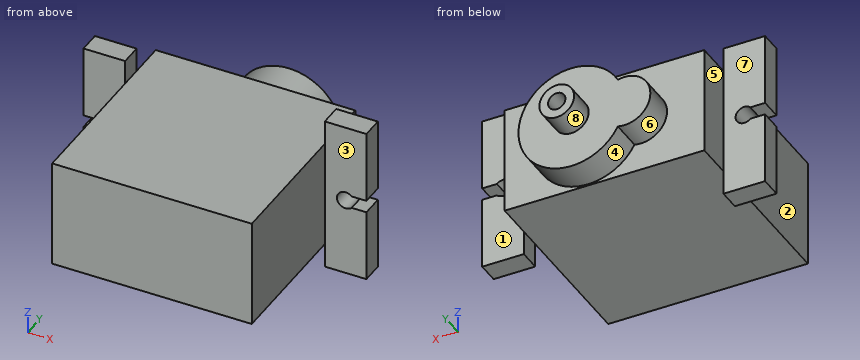
Autodesk Inventor part; units mm, degrees
ref_plane "Work Plane3" through (-11.5, 0, 0) normal (1, 0, 0) x (0, 1, 0)
ref_plane "Work Plane4" through (0, 5, 0) normal (0, 1, 0) x (-1, 0, 0)
ref_plane "Work Plane5" through (0, 0, 6.25) normal (0, 0, 1) x (1, 0, 0)
sketch "Sketch1" plane through (0, 0, 0) normal (0, 1, 0) x (-1, 0, 0)
  line L0 (11.5, -6.25) -> (-11.5, -6.25)
  line L1 (-11.5, -6.25) -> (-11.5, 6.25)
  line L2 (-11.5, 6.25) -> (11.5, 6.25)
  line L3 (11.5, 6.25) -> (11.5, -6.25)
  line L4 (11.5, -6.25) -> (-11.5, 6.25) construction
  line L5 (-11.5, -6.25) -> (11.5, 6.25) construction
  point P0 (0, 0)
  dimension "d0" = 23
  dimension "d1" = 12.5
extrude "Extrusion1" add sketch "Sketch1" along normal mid plane 22.7
ref_plane "Work Plane3" through (-11.5, 0, 0) normal (1, 0, 0) x (0, 1, 0)
ref_plane "Work Plane2" through (11.5, 0, 0) normal (1, 0, 0) x (0, 1, 0)
ref_plane "Work Plane4" through (0, 5, 0) normal (0, 1, 0) x (-1, 0, 0)
ref_plane "Work Plane5" through (0, 0, 6.25) normal (0, 0, 1) x (1, 0, 0)
sketch "Sketch2" plane through (11.5, -11.35, -6.25) normal (1, 0, 0) x (0, 0, -1)
  line L0 (0, 0) -> (-12.5, 0)
  line L1 (-12.5, 0) -> (-12.5, 16)
  line L2 (-12.5, 0) -> (-12.5, 22.7)
  line L3 (-12.5, 16) -> (-15.3, 16)
  line L4 (-15.3, 16) -> (-15.3, 18.5)
  line L5 (-15.3, 18.5) -> (0, 18.5)
  line L6 (0, 18.5) -> (2.8, 18.5)
  line L7 (2.8, 18.5) -> (2.8, 16)
  line L8 (2.8, 16) -> (-12.5, 16)
  point P0 (-6.25, 11.35)
  dimension "d8" = 16
  dimension "d9" = 2.8
  dimension "d10" = 2.5
  dimension "d11" = 2.8
extrude "Extrusion2" add sketch "Sketch2" along normal blind 4.8
mirror "Mirror1" about plane through (0, 0, 0) normal (1, 0, 0) of "Extrusion2"
ref_plane "Work Plane6" through (0, 11, 0) normal (0, 1, 0) x (-1, 0, 0)
sketch "Sketch3" plane through (0, 11, 0) normal (0, 1, 0) x (-1, 0, 0)
  line L0 (-12.5008, 0) -> (-1.9008, 0)
  arc A0 (3.4585, 2.9134) -> (3.4585, -2.9134) centre (-1.9008, 0) ccw
  circle A1 centre (-1.9008, 0) radius 1
  arc A2 (3.4585, -2.9134) -> (3.4585, 2.9134) centre (4.1992, 0) ccw
  point P0 (0, 0)
  dimension "d15" = 10.6
  dimension "d16" = 12.2
  dimension "d17" = 2
extrude "Extrusion3" add sketch "Sketch3" along normal blind 4
sketch "Sketch4" plane through (0, 15, 0) normal (0, 1, 0) x (1, 0, 0)
  circle A0 centre (1.9008, 0) radius 1
  circle A1 centre (1.9008, 0) radius 2
  point P0 (0, 0)
  dimension "d20" = 4
extrude "Extrusion4" add sketch "Sketch4" along normal blind 3.2 contours A0 | A1
sketch "Sketch5" plane through (1.9008, 18.2, 0) normal (0, 1, 0) x (1, 0, 0)
  circle A0 centre (0, 0) radius 1
  circle A1 centre (0, 0) radius 1
  point P0 (-1.9008, 0)
  dimension "d28" = 2
extrude "Extrusion5" cut sketch "Sketch5" against normal blind 3.2
sketch "Sketch6" plane through (11.5, 7.15, -6.25) normal (0, 1, 0) x (1, 0, 0)
  circle A0 centre (-9.5992, -6.25) radius 1
  line L0 (-9.5992, -6.25) -> (1.4, -6.25)
  line L1 (4.8, -15.3) -> (4.8, 2.8)
  line L2 (0, -12.5) -> (0, 0)
  line L3 (0, -6.25) -> (4.8, -6.25)
  arc A1 (3.1037, -5.5395) -> (3.1037, -6.9605) centre (2.4, -6.25) ccw
  line L4 (2.4, -5.25) -> (2.4, -5.25)
  line L5 (3.1037, -5.5395) -> (4.8, -5.5395)
  line L6 (3.1037, -6.9605) -> (4.8, -6.9605)
  line L7 (4.8, -6.9605) -> (4.8, -5.5395)
  point P0 (-11.5, -6.25)
  dimension "d25" = 2
extrude "Extrusion6" cut sketch "Sketch6" against normal blind 2.5 contours A1 L5 L1 L3 | L3 L1 L6 A1
mirror "Mirror2" about plane through (0, 0, 0) normal (1, 0, 0) of "Extrusion6"
properties part number "Motor"
Build history of the part. All positions in model axes, mm. Face numbers are marked on the shaded views. A direction names the side the tool comes from. Coordinates: 2 decimals unless noted, no trailing zeros. Order: outer loops, then holes, each group sorted by start corner. A loop starts at its lowest first (then second) coordinate and runs counter-clockwise, first axis right, second up. Notation, with made-up numbers: M -24,-19 L -5,-19 A30 ccw -5,17 Z; hole C -20.75,12.5 d1. An arc over 180 degrees is marked long. One line per question, with ' | ' between items. Start each with the question number.
Q1. Saw through at A-A (z = 8). List the corners of the cut face in (x, y), then the cut area to 3 significant figures.
Q2. Saw through at C-C (z = 0). List the corners of the cut face in (x, y), then the cut area to 3 significant figures.
Q3. Flat gauge pins, fed straight in: pin 1 Ø8 at (x, z) = (-5.5, 4.5) entering from +Y; pin 2 Ø3 at (y, z) = (2.5, -3.5) entering from -X; pin 3 Ø8 at (x, z) = (-13, -4) entering from +Y. Where does each tip first touch, or does it go through?
Q4. 3-axis set-ups, long thin cutter, end or side, ignore diameter. For the marked faces 1, 2, 3, 4 and 5: which of +Z, -Z, +X, -X, +Y, -Y reach the whole face in a straight line?
Q5. Probe L1, parallel to Z at x = 13.9, y = 6.5; L2, parallel to Y at x = 12, z = -5.5; L3, parallel to Y at x = 10.5, z = 5.5. List the from-to ranges inside material, lowest first. Write a range as from..to.
Q6. Two-plate mould, pull along X, no slides. Class the marked faces 6, 7 and 8: +X half, -X half, draft (parallel to the pull), parting line (faces both ways), or undercut.
Q7. Saw through at B-B (x = -13.9). List the corners of the cut face in (y, z), then the cut area to 4 significant figures.
Q8. Saw through at D-D (x = -1.5). List the corners of the cut face in (y, z).
Check values:
1) outline: M -16.3,4.65 L -11.5,4.65 L -11.5,7.15 L -16.3,7.15 Z; M 11.5,4.65 L 16.3,4.65 L 16.3,7.15 L 11.5,7.15 Z | area: 24.0 mm2
2) outline: M -12.9,4.65 L -11.5,4.65 L -11.5,-11.35 L 11.5,-11.35 L 11.5,4.65 L 12.9,4.65 L 12.9,7.15 L 11.5,7.15 L 11.5,11.35 L 8,11.35 L 8,15 L 3.9,15 L 3.9,18.2 L 2.9,18.2 L 2.9,11.35 L 0.9,11.35 L 0.9,18.2 L -0.1,18.2 L -0.1,15 L -7.21,15 L -7.21,11.35 L -11.5,11.35 L -11.5,7.15 L -12.9,7.15 Z | area: 584 mm2
3) pin 1: stops at y = 15 | pin 2: stops at x = -11.5 | pin 3: stops at y = 11.35
4) face 1: +Z, -Z, +X, +Y | face 2: +Z, -Z, -X, -Y | face 3: +Z, -Z, +X, -Y | face 4: +Y | face 5: +Z, -Z, -X, +Y
5) L1: z = -9.05..-1, 1..9.05 | L2: y = 4.65..7.15 | L3: y = -11.35..11.35
6) face 6: undercut | face 7: draft | face 8: parting line
7) outline: M 4.65,-9.05 L 7.15,-9.05 L 7.15,-1 L 4.65,-1 Z; M 4.65,1 L 7.15,1 L 7.15,9.05 L 4.65,9.05 Z | area: 40.25 mm2
8) outline: M -11.35,-6.25 L 11.35,-6.25 L 11.35,-5.06 L 15,-5.06 L 15,5.06 L 11.35,5.06 L 11.35,6.25 L -11.35,6.25 Z
